Here's the drawing with two shaded views (mm, measured from the low corner). I have some questions. A direction names the side the tool comes from. Give positions to 0.01 mm unless a question says otherwise; leave off trailing zeros. Write each loop counter-clockwise with the first axis right and the second up, starting at its lowest first coordinate (ties: lowest second). Pieces come first, ordered by that corner, then holes. Notation, with made-up numbers: M 80.5,41 L 130.5,41 A27 ccw 130.5,80 Z; hole C 5,35.25 d8. An arc over 180 degrees is marked long. Use one line per item in the form item = value.
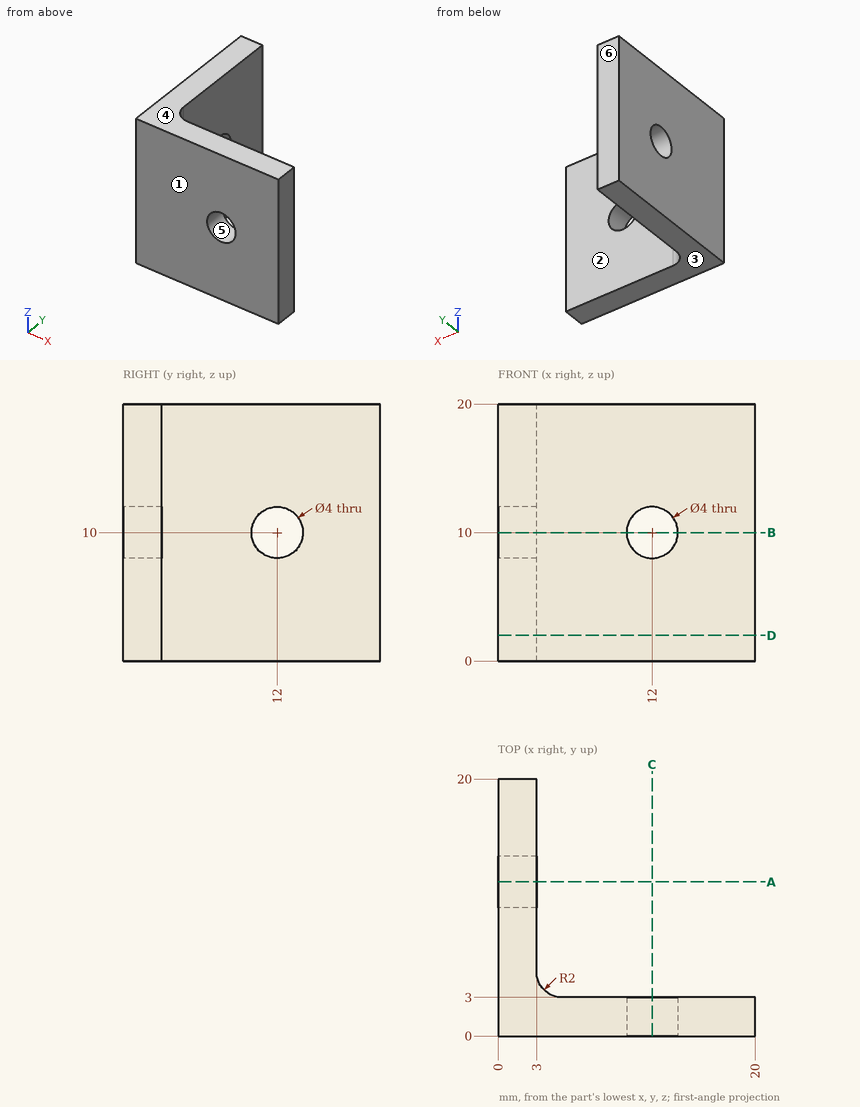
1) For pin 1 Ø1 at (y, z) = (5, 13) entering from +X; pin 2 Ø6 at (x, y) = (8, 8.5) entering from -Z; pin 3 Ø5 at (x, z) = (10, 8.5) entering from +Y, each with a flat end and sliding along its axis, tell me the tip position at first contact or that it passes through.
Checked values:
pin_1 = 3.06
pin_2 = through
pin_3 = 3
2) I want a section at B-B, the plane z = 10. Please give me the cut outline in (x, y), plus the area to 3 significant figures.
Checked values:
outline = M 0,0 L 10,0 L 10,3 L 5,3 A2 cw 3,5 L 3,10 L 0,10 Z; M 0,14 L 3,14 L 3,20 L 0,20 Z; M 14,0 L 20,0 L 20,3 L 14,3 Z
area = 87.9 mm2
3) For the marked faces 1 and 2, which set-ups out of +Z, -Z, +X, -X, +Y, -Y let a thin tool reach every point of the face, with its end or its side?
Checked values:
face_1 = +Z, -Z, +X, -X, -Y
face_2 = +Z, -Z, +X, +Y
4) Thinking about a two-plate mould opening in Z: for the marked faces 3, 4, 5 and 6, which applies, released by +Z, released by -Z, zero draft, split by the parting line, or undercut?
Checked values:
face_3 = released by -Z
face_4 = released by +Z
face_5 = undercut
face_6 = zero draft
5) I want a section at D-D, the plane z = 2. Please give me the cut outline in (x, y), plus the area to 3 significant figures.
Checked values:
outline = M 0,0 L 20,0 L 20,3 L 5,3 A2 cw 3,5 L 3,20 L 0,20 Z
area = 112 mm2
6) I want a section at A-A, the plane y = 12. Please give me the cut outline in (x, z).
Checked values:
outline = M 0,0 L 3,0 L 3,8 L 0,8 Z; M 0,12 L 3,12 L 3,20 L 0,20 Z
7) If I drill on L1, parallel to Z at x = 12, y = 1.65; L2, parallel to Y at x = 1.4, z = 10, over which ranges is the centre line in solid material (lowest first)?
Checked values:
L1 = 0 to 8, 12 to 20
L2 = 0 to 10, 14 to 20
